Build history of the part. All positions in model axes, mm. A direction names the side the tool comes from. Give positions to 0.01 mm unless a question says otherwise; leave off trailing zeros. Write each loop counter-clockwise with the first axis right and the second up, starting at its lowest first coordinate (ties: lowest second). Pieces come first, ordered by that corner, then holes. Notation, with made-up numbers: M 20,57.25 L 58,57.25 A37 ccw 58,93.25 Z; hole C 34,46.5 d10. An arc over 180 degrees is marked long. Return JSON: item names as keys, results as strings. Group by question number.
Q1. Tool access for faces 5 (the flat face through (22.611, 4.701, -34.323)), 6 (the flat face through (22.75, 0.196, -34.469)), 7 (the flat face through (22.75, 9.33, -34.47)), 8 (the flat face through (-6.35, 5, -27)), 9 (the flat face through (-3.333, 4.701, -76.458)): list every direction of +Z, -Z, +X, -X, +Y, -Y with a clear straight run to the whole face (end or side of a thin tool).
Q2. Flat gauge pins, fed straight in: pin 1 Ø2.5 at (x, z) = (13.73, -51.51) entering from +Y; pin 2 Ø5 at (x, y) = (27.5, 5.5) entering from +Z; pin 3 Ø4.5 at (x, y) = (22, 3.5) entering from -Z; pin 4 Ø1.5 at (y, z) = (7.5, -58.5) entering from -X. Where does each tip first touch, or does it go through?
Q3. Wall check: probe 1 along X at (y, z) = (3.25, -12.7); probe 2 along Z at (x, y) = (0, 5.75); probe 3 along X at (y, z) = (7, -127). Give the ranges that are in metal, low to high.
Q4. Band-saw the part on B-B, the plane y = 5.75. Count the separate pieces of the cut face and the enclosed holes in it, then the cut area to 3 significant figures.
Q5. Band-saw the part on D-D, the plane x = -63.5. Give the cut face in (y, z) (1 decimal), then the cut area to 3 significant figures.
Q6. Band-saw the part on C-C, the plane z = -127. Give the cut face in (x, y) (1 decimal).
Q7. Band-saw the part on A-A, the plane z = -12.7. Give the cut face in (x, y) (3 decimals), then the cut area to 3 significant figures.
Q8. Pull direction X, two halves, no side cores. Call faces 1 (the cylindrical face through (56.62, 4.7, -18.86)), 2 (the flat face through (4, 0, -48)), 3 (the conical face through (-66.701, 9.418, -130.124)), 4 (the cylindrical face through (-65.109, 4.701, -128.475)): +X half, -X half, draft (parallel to the pull), parting line (faces both ways), or undercut.
from build123d import *

# Parameters (mm, degrees)
SKETCH1_R           = 2.1828125
BOSS_EXTRUDE1_DEPTH = 9.525
CHAMFER1_SIZE       = 0.396875


with BuildPart() as part:
    # Sketch1 → Boss-Extrude1 (new body)
    with BuildSketch(Plane(origin=(0, 0, 0), x_dir=(1, 0, 0), z_dir=(0, 1, 0))):
        with BuildLine():
            Line((-6.35, 0), (-6.35, 54.968986339))
            ThreePointArc((-6.35, 54.968986339), (-6.780470884, 57.267175854), (-8.013519701, 59.253773662))
            Line((-8.013519701, 59.253773662), (-67.014860224, 123.786409508))
            ThreePointArc((-67.014860224, 123.786409508), (-66.836015353, 130.398883319), (-60.221355188, 130.454257437))
            Line((-60.221355188, 130.454257437), (55.171526417, 20.927889031))
            ThreePointArc((55.171526417, 20.927889031), (56.634453391, 18.828535178), (57.15, 16.322212447))
            Line((57.15, 16.322212447), (57.15, 0))
            ThreePointArc((57.15, 0), (55.290128061, -4.490128061), (50.8, -6.35))
            ThreePointArc((50.8, -6.35), (46.309797545, -4.490202455), (44.45, -0.000254))
            ThreePointArc((44.45, -0.000254), (42.590202455, 4.490202455), (38.100254, 6.35))
            Line((38.100254, 6.35), (12.699746, 6.35))
            ThreePointArc((12.699746, 6.35), (8.209797545, 4.490202455), (6.35, 0.000254))
            ThreePointArc((6.35, 0.000254), (4.490202455, -4.490202455), (0.000254, -6.35))
            ThreePointArc((0.000254, -6.35), (-4.490128061, -4.490128061), (-6.35, 0))
        make_face()
        Circle(SKETCH1_R, mode=Mode.SUBTRACT)
        with Locations((50.8, 12.7)):
            Circle(SKETCH1_R, mode=Mode.SUBTRACT)
        with Locations((-63.5, 127)):
            Circle(SKETCH1_R, mode=Mode.SUBTRACT)
        with Locations((0, 12.7)):
            Circle(SKETCH1_R, mode=Mode.SUBTRACT)
        with Locations((50.8, 0)):
            Circle(SKETCH1_R, mode=Mode.SUBTRACT)
        with Locations((13.727904726, 51.509581964)):
            Circle(SKETCH1_R, mode=Mode.SUBTRACT)
        with BuildLine():
            Line((35.81658762, 21.788919146), (9.030381604, 47.213328586))
            ThreePointArc((9.030381604, 47.213328586), (7.310919317, 47.520522788), (6.35, 46.06190944))
            Line((6.35, 46.06190944), (6.35, 20.6375))
            ThreePointArc((6.35, 20.6375), (6.814967985, 19.514967985), (7.9375, 19.05))
            Line((7.9375, 19.05), (34.723706016, 19.05))
            ThreePointArc((34.723706016, 19.05), (36.198160855, 20.04916406), (35.81658762, 21.788919146))
        make_face(mode=Mode.SUBTRACT)
    extrude(amount=BOSS_EXTRUDE1_DEPTH)

    # Chamfer1
    chamfer1_edges = [part.edges().sort_by_distance(p)[0] for p in [
        (56.634453391, 9.525, -18.828535178),
        (-2.524914386, 9.525, -75.691073234),
        (46.309887349, 0, 4.490292258),
        (46.309887349, 0, 4.490292258),
        (42.59038206, 0, -4.490022844),
        (42.59038206, 0, -4.490022844),
        (25.4, 0, -6.35),
        (8.209797545, 0, -4.490202455),
        (4.49038206, 0, 4.490022844),
        (4.49038206, 0, 4.490022844),
        (-4.490038256, 0, 4.490217863),
        (-66.836015353, 9.525, -130.398883319),
        (-4.490038256, 0, 4.490217863),
        (-6.35, 0, -27.484493169),
        (-6.780470884, 0, -57.267175854),
        (-37.514189963, 0, -91.520091585),
        (-66.836015353, 0, -130.398883319),
        (-2.524914386, 0, -75.691073234),
        (56.634453391, 0, -18.828535178),
        (57.15, 0, -8.161106224),
        (55.290128061, 0, 4.490128061),
        (-37.514189963, 9.525, -91.520091585),
        (-6.780470884, 9.525, -57.267175854),
        (-6.35, 9.525, -27.484493169),
        (-4.490038256, 9.525, 4.490217863),
        (-4.490038256, 9.525, 4.490217863),
        (-2.1828125, 0, 0),
        (4.49038206, 9.525, 4.490022844),
        (-2.1828125, 9.525, 0),
        (48.6171875, 0, -12.7),
        (48.6171875, 9.525, -12.7),
        (4.49038206, 9.525, 4.490022844),
        (55.290128061, 9.525, 4.490128061),
        (-65.6828125, 0, -127),
        (-65.6828125, 9.525, -127),
        (8.209797545, 9.525, -4.490202455),
        (-2.1828125, 0, -12.7),
        (-2.1828125, 9.525, -12.7),
        (25.4, 9.525, -6.35),
        (48.6171875, 0, 0),
        (48.6171875, 9.525, 0),
        (42.59038206, 9.525, -4.490022844),
        (42.59038206, 9.525, -4.490022844),
        (36.198160855, 0, -20.04916406),
        (22.423484612, 0, -34.501123866),
        (7.310919317, 0, -47.520522788),
        (46.309887349, 9.525, 4.490292258),
        (6.35, 0, -33.34970472),
        (6.814967985, 0, -19.514967985),
        (21.330603008, 0, -19.05),
        (36.198160855, 9.525, -20.04916406),
        (22.423484612, 9.525, -34.501123866),
        (7.310919317, 9.525, -47.520522788),
        (6.35, 9.525, -33.34970472),
        (6.814967985, 9.525, -19.514967985),
        (21.330603008, 9.525, -19.05),
        (46.309887349, 9.525, 4.490292258),
        (11.545092226, 0, -51.509581964),
        (11.545092226, 9.525, -51.509581964),
        (57.15, 9.525, -8.161106224),
    ]]
    chamfer(chamfer1_edges, length=CHAMFER1_SIZE)


solid = part.part
From the geometry:
{
 "1": {"face 5": "+Y, -Y", "face 6": "-Y", "face 7": "+Y", "face 8": "+Z, -X, +Y, -Y", "face 9": "-Z, +X, +Y, -Y"},
 "2": {"pin 1": "passes through", "pin 2": "stops at z = -6.35", "pin 3": "stops at z = -54.55", "pin 4": "stops at x = -8.01"},
 "3": {"probe 1": "x = -6.35 to -2.18, 2.18 to 48.62, 52.98 to 57.15", "probe 2": "z = -73.29 to -14.88, -10.52 to -2.18, 2.18 to 6.35", "probe 3": "x = -68.26 to -65.68, -61.32 to -56.58"},
 "4": {"separate pieces": "1", "enclosed holes": "7", "area": "3,500 mm^2"},
 "5": {"outline": "M 0,-131.4 L 0.4,-131.8 L 9.1,-131.8 L 9.5,-131.4 L 9.5,-129.6 L 9.1,-129.2 L 0.4,-129.2 L 0,-129.6 Z; M 0,-124.4 L 0.4,-124.8 L 9.1,-124.8 L 9.5,-124.4 L 9.5,-120.5 L 9.1,-119.9 L 0.4,-119.9 L 0,-120.5 Z", "area": "70.3 mm^2"},
 "6": {"outline": "M -68.3,0.4 L -67.9,0 L -66.1,0 L -65.7,0.4 L -65.7,9.1 L -66.1,9.5 L -67.9,9.5 L -68.3,9.1 Z; M -61.3,0.4 L -60.9,0 L -57.2,0 L -56.6,0.4 L -56.6,9.1 L -57.2,9.5 L -60.9,9.5 L -61.3,9.1 Z"},
 "7": {"outline": "M -6.35,0.397 L -5.953,0 L -2.58,0 L -2.183,0.397 L -2.183,9.128 L -2.58,9.525 L -5.953,9.525 L -6.35,9.128 Z; M 2.183,0.397 L 2.58,0 L 48.22,0 L 48.617,0.397 L 48.617,9.128 L 48.22,9.525 L 2.58,9.525 L 2.183,9.128 Z; M 52.983,0.397 L 53.38,0 L 56.753,0 L 57.15,0.397 L 57.15,9.128 L 56.753,9.525 L 53.38,9.525 L 52.983,9.128 Z", "area": "521 mm^2"},
 "8": {"face 1": "+X half", "face 2": "draft", "face 3": "parting line", "face 4": "undercut"}
}
